Autodesk Inventor part; units mm, degrees
ref_plane "РабПлоскость1" through (17.5, 36.1, 84) normal (0, 1, 0) x (1, 0, 0)
ref_plane "YZ Plane" through (0, 0, 0) normal (1, 0, 0) x (0, 1, 0)
ref_plane "XZ Plane" through (0, 0, 0) normal (0, 1, 0) x (-1, 0, 0)
sketch "Эскиз1" plane through (0, 0, 0) normal (0, 1, 0) x (-1, 0, 0)
  arc A0 (6.0208, -6) -> (6.0208, 6) centre (0, 0) ccw
  line L0 (6.0208, -6) -> (-6.0208, -6)
  arc A1 (-6.0208, 6) -> (-6.0208, -6) centre (0, 0) ccw
  line L1 (6.0208, 6) -> (-6.0208, 6)
  line L2 (17.5, 37) -> (-17.5, 37)
  line L3 (-17.5, 37) -> (-17.5, 0)
  arc A2 (-17.5, 0) -> (17.5, 0) centre (0, 0) ccw
  line L4 (17.5, 0) -> (17.5, 37)
  line L5 (17.5, 0) -> (17.5, 57)
  line L6 (-17.5, 37) -> (17.5, 37)
  line L7 (17.5, 37) -> (17.5, 57)
  line L8 (17.5, 57) -> (-17.5, 57)
  line L9 (-17.5, 57) -> (-17.5, 37)
extrude "Выдавливание1" add sketch "Эскиз1" along normal blind 27
sketch "Эскиз2" plane through (-17.5, 0, 57) normal (0, 0, 1) x (1, 0, 0)
  line L0 (0, 0) -> (35, 0)
  line L1 (35, 0) -> (35, 72.2)
  line L2 (35, 72.2) -> (0, 72.2)
  line L3 (0, 72.2) -> (0, 0)
  point P0 (17.5, 0)
  dimension "d2" = 72.2
extrude "Выдавливание2" add sketch "Эскиз2" along normal blind 27
ref_plane "РабПлоскость1" through (17.5, 36.1, 84) normal (0, 1, 0) x (1, 0, 0)
mirror "Зеркальное отражение1" about plane through (17.5, 36.1, 84) normal (0, 1, 0) of "Выдавливание1"
sketch "Эскиз3" plane through (17.5, 0, 0) normal (1, 0, 0) x (0, 0, -1)
  line L0 (-57, 45.2) -> (-57, 27)
  line L1 (-57, 36.1) -> (-42, 36.1)
  circle A0 centre (-42, 36.1) radius 18
  point P0 (0, 0)
  dimension "d5" = 15
  dimension "d6" = 36
extrude "Выдавливание3" cut sketch "Эскиз3" against normal blind 93.5
chamfer "Фаска2" distance 8 angle 45 8 edges at (0, 27, 26.4697) (0, 45.2, 26.4697) (-17.5, 27, 13.2349) (0, 27, -17.5) (17.5, 27, 13.2349) (-17.5, 45.2, 13.2349) (0, 45.2, -17.5) (17.5, 45.2, 13.2349)
move faces "Перенос1" translate (0, 0, 18) faces at (-5.8333, 48.1333, 84)
sketch "Эскиз4" plane through (17.5, 36.1, 42) normal (1, 0, 0) x (0, 0, -1)
  line L0 (-60, -36.1) -> (-60, 36.1)
  line L1 (-60, 0) -> (-45, 0)
  line L2 (-52.5, -15) -> (-37.5, -15)
  line L3 (-37.5, -15) -> (-37.5, 15)
  line L4 (-37.5, 15) -> (-52.5, 15)
  line L5 (-52.5, 15) -> (-52.5, -15)
  line L6 (-52.5, -15) -> (-37.5, 15) construction
  line L7 (-37.5, -15) -> (-52.5, 15) construction
  point P0 (42, -36.1)
  dimension "d18" = 15
  dimension "d19" = 15
  dimension "d20" = 30
extrude "Выдавливание4" cut sketch "Эскиз4" against normal blind 79.25
sketch "Эскиз5" plane through (-17.5, 0, 102) normal (0, 0, 1) x (1, 0, 0)
  line L0 (23.5208, 72.2) -> (11.4792, 72.2)
  line L1 (17.5, 72.2) -> (17.5, 36.1)
  circle A0 centre (17.5, 36.1) radius 10
  point P0 (17.5, 0)
  dimension "d23" = 36.1
  dimension "d24" = 20
extrude "Выдавливание5" cut sketch "Эскиз5" against normal blind 12.5
sketch "Эскиз14" plane through (-17.5, 0, 102) normal (0, 0, 1) x (1, 0, 0)
  circle A0 centre (17.5, 36.1) radius 10
  line L0 (17.5, 36.1) -> (17.5, 61.1)
  circle A1 centre (17.5, 61.1) radius 1.9
  line L1 (17.5, 36.1) -> (17.5, 11.1)
  circle A2 centre (17.5, 11.1) radius 1.9
  point P0 (17.5, 0)
  dimension "d47" = 25
  dimension "d48" = 3.8
  dimension "d49" = 25
  dimension "d50" = 3.8
extrude "Выдавливание13" cut sketch "Эскиз14" against normal blind 20.35 contours A1 | A2
sketch "Эскиз15" plane through (-17.5, 0, 102) normal (0, 0, 1) x (1, 0, 0)
  circle A0 centre (17.5, 61.1) radius 1.9
  circle A1 centre (17.5, 11.1) radius 1.9
  circle A2 centre (17.5, 36.1) radius 10
  line L0 (0, 0) -> (35, 0)
  line L1 (35, 0) -> (35, 72.2)
  line L2 (35, 72.2) -> (0, 72.2)
  line L3 (0, 72.2) -> (0, 0)
  point P0 (17.5, 0)
properties part number "joint_2_part1" material "Пластик АБС"
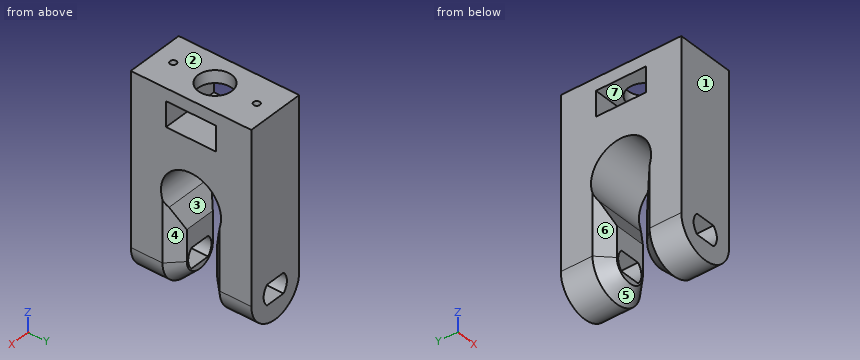
Here's how the part is built. I have some questions about the finished solid (model axes, mm). Face numbers are marked on the shaded views. A direction names the side the tool comes from. Give positions to 0.01 mm unless a question says otherwise; leave off trailing zeros. Order: outer loops, then holes, each group sorted by start corner. A loop starts at its lowest first (then second) coordinate and runs counter-clockwise, first axis right, second up. Notation, with made-up numbers: (-17.75, 5) - (28.25, 5) arc R11 ccw to (28.25, 17) - close; hole circle Ø6 at (4, -10). An arc over 180 degrees is marked (long way). Answer as a JSON object with one key per item and string values. Group by question number.
Item 1: If we section it at A-A on z = 42: Please give me the cut outline in (x, y).
Item 2: Which directions (+Z, -Z, +X, -X, +Y, -Y) give clear straight access to the entire face, cutting with the end or side of a thin tool? Please do the marked faces 4, 5, 6 and 7.
Item 3: Please list where these lines run through material, in increasing order: probe 1 along Y at (x, z) = (0, 98); probe 2 along Y at (x, z) = (0, 91); probe 3 along X at (y, z) = (5, 0).
Item 4: If we section it at B-B on y = 36.1: Please give me the cut outline in (x, z).
Item 5: If we section it at D-D on x = 0: Give the number of separate pieces and of enclosed holes in the cut face, and give its area (3 significant figures).
Item 6: If we mould it in two halves opening along Y, with no side actions, what happens to the marked faces 1, 2 and 3? For each: pulls with the +Y half, pulls with the -Y half, needs draft (parallel to the pull), parting line crosses it, or undercut.
Item 7: If we section it at C-C on y = 11.1: Please give me the cut outline in (x, z).
Item 8: For P1, Ø1.1, axis at x = -0.5, y = 61, coming from the +Z side; P2, Ø5, axis at x = 9, y = 41, coming from the -Z side; P3, Ø3, axis at x = -8.5, y = 47, coming from the -Z side, each with a flat end and sliding along its axis, tell me the tip position at first contact or that it passes through.
Result set:
{
 "1": {"outline": "(-17.5, 0) - (17.5, 0) - (17.5, 18.1) - (-17.5, 18.1) - close; (-17.5, 54.1) - (17.5, 54.1) - (17.5, 72.2) - (-17.5, 72.2) - close"},
 "2": {"face 4": "-Z, +X", "face 5": "-Z", "face 6": "-Z, -X", "face 7": "+X, -X"},
 "3": {"probe 1": "0 to 9.2, 13 to 26.1, 46.1 to 59.2, 63 to 72.2", "probe 2": "0 to 9.2, 13 to 21.1, 51.1 to 59.2, 63 to 72.2", "probe 3": "-17.5 to -8.5, 8.5 to 17.5"},
 "4": {"outline": "(-17.5, 60) - (17.5, 60) - (17.5, 79.5) - (-17.5, 79.5) - close; (-17.5, 94.5) - (-10, 94.5) - (-10, 102) - (-17.5, 102) - close; (10, 94.5) - (17.5, 94.5) - (17.5, 102) - (10, 102) - close"},
 "5": {"separate pieces": "3", "enclosed holes": "0", "area": "5,330 mm²"},
 "6": {"face 1": "pulls with the -Y half", "face 2": "needs draft", "face 3": "undercut"},
 "7": {"outline": "(-17.5, 0) arc R17.5 ccw to (17.5, 0) - (17.5, 102) - (1.9, 102) - (1.9, 81.65) - (-1.9, 81.65) - (-1.9, 102) - (-17.5, 102) - close; hole (-6.02, -6) - (6.02, -6) arc R8.5 ccw to (6.02, 6) - (-6.02, 6) arc R8.5 ccw to start"},
 "8": {"P1": "z = 81.65", "P2": "z = 58.41", "P3": "z = -9.93"}
}
